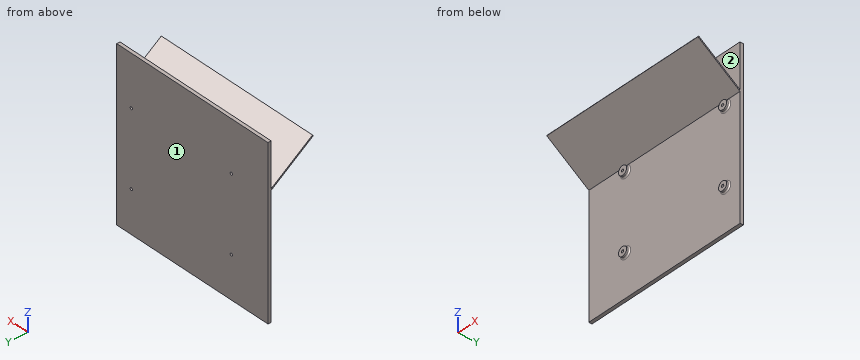
Autodesk Inventor part; units mm, degrees
ref_plane "YZ Plane" through (0, 0, 0) normal (1, 0, 0) x (0, 1, 0)
ref_plane "XZ Plane" through (0, 0, 0) normal (0, 1, 0) x (-1, 0, 0)
ref_plane "XY Plane" through (0, 0, 0) normal (0, 0, 1) x (1, 0, 0)
sketch "Sketch1" plane through (0, 0, 0) normal (0, 1, 0) x (-1, 0, 0)
  line L0 (0, 0) -> (130, 0)
  line L1 (130, 0) -> (130, -130)
  line L2 (130, -130) -> (0, -130)
  line L3 (0, -130) -> (0, 0)
  dimension "d0" = 130
  dimension "d1" = 130
extrude "Extrusion1" add sketch "Sketch1" along normal blind 2.5
sketch "Sketch2" plane through (0, 0, 0) normal (0, -1, 0) x (1, 0, 0)
  line L0 (-2.5, -114.4468) -> (-102.5, -114.4468) construction
  line L1 (-102.5, -114.4468) -> (-102.5, -35.4468) construction
  line L2 (-102.5, -35.4468) -> (-2.5, -35.4468) construction
  line L3 (-2.5, -35.4468) -> (-2.5, -114.4468) construction
  line L4 (-12.5, -97.4468) -> (-98.5, -97.4468) construction
  line L5 (-98.5, -97.4468) -> (-98.5, -39.4468) construction
  line L6 (-98.5, -39.4468) -> (-12.5, -39.4468) construction
  line L7 (-12.5, -39.4468) -> (-12.5, -97.4468) construction
  line L8 (0, 0) -> (-130, 0) construction
  line L9 (-130, -130) -> (0, -130) construction
  line L10 (-130, 0) -> (-130, -130) construction
  circle A0 centre (-12.5, -97.4468) radius 3.5
  circle A1 centre (-98.5, -97.4468) radius 3.5
  circle A2 centre (-12.5, -39.4468) radius 3.5
  circle A3 centre (-98.5, -39.4468) radius 3.5
  line L11 (0, -130) -> (0, 0)
  line L12 (-91.6778, -53.8) -> (-93.3369, -53.8) construction
  line L13 (-93.3369, -53.8) -> (-93.3369, -76.2) construction
  line L14 (-93.3369, -76.2) -> (-91.6778, -76.2) construction
  line L15 (-91.6778, -76.2) -> (-91.6778, -53.8) construction
  dimension "d4" = 86
  dimension "d5" = 58
  dimension "d6" = 100
  dimension "d7" = 79
  dimension "d8" = 4
  dimension "d9" = 4
  dimension "d10" = 130
  dimension "d13" = 7
  dimension "d14" = 7
  dimension "d15" = 7
  dimension "d16" = 7
  dimension "d27" = 2.5
  dimension "d34" = 22.4
  dimension "d35" = 21.2468
  dimension "d36" = 53.8
extrude "Extrusion2" add sketch "Sketch2" along normal blind 2.25
fillet "Fillet1" radius 1 4 edges at (-16, 0, -97.4468) (-16, 0, -39.4468) (-102, 0, -39.4468) (-102, 0, -97.4468)
sketch "Sketch3" plane through (-12.5, -2.25, -97.4468) normal (0, -1, 0) x (1, 0, 0)
  circle A0 centre (0, 0) radius 3.5 construction
  circle A1 centre (-86, 0) radius 3.5 construction
  circle A2 centre (0, 58) radius 3.5 construction
  circle A3 centre (-86, 58) radius 3.5 construction
  circle A4 centre (0, 0) radius 4.5 construction
  circle A5 centre (-86, 58) radius 3.5 construction
  point P0 (12.5, 97.4468)
  point P1 (0, 58)
  point P2 (-86, 58)
  point P3 (-86, 0)
hole "Hole1" at (-12.5, -2.25, -97.4468) at (-12.5, -2.25, -39.4468) at (-98.5, -2.25, -39.4468) at (-98.5, -2.25, -97.4468) direction (0, 1, 0) diameter 2.013 depth 4.75
sketch "Sketch4" plane through (0, 0, 0) normal (1, 0, 0) x (0, 0, -1)
  line L0 (130, 0) -> (0, 0)
  line L1 (35.4468, 0) -> (1.8296, -48.0104) construction
  line L2 (35.4468, 0) -> (12.5038, -32.7661)
  line L3 (12.5038, -32.7661) -> (11.6846, -32.1925)
  line L4 (11.6846, -32.1925) -> (34.2261, 0)
  line L5 (35.4468, 0) -> (34.2261, 0)
  point P0 (35.4468, 0)
  dimension "d28" = 55
  dimension "d29" = 0
  dimension "d30" = 1
  dimension "d31" = 40
extrude "Extrusion3" add sketch "Sketch4" against normal blind 130
sketch "Sketch5" plane through (0, 2.5, 0) normal (1, 0, 0) x (0, 0, -1)
  line L0 (34.2261, -2.5) -> (11.6846, -34.6925)
  point P0 (0, -2.5)
equation "\"d9\" = d8"
equation "\"d14\" = d13"
equation "\"d15\" = d14"
equation "\"d16\" = d15"
equation "\"d36\" = -0.5 * d34 + 0.5 * d10"
properties part number "angle test"
Verification items for the finished model (mm, model axes). Face numbers are marked on the shaded views. A direction names the side the tool comes from. Give positions to 0.01 mm unless a question says otherwise; leave off trailing zeros. Loops run counter-clockwise (first coordinate to the right, second up) from the corner with the lowest first, then second, coordinate; pieces in that order, holes last. Notation, with made-up numbers: (62.25, 81) - (85.25, 81) arc R28 cw to (85.25, 107) - close; hole circle Ø9 at (-23.5, 32.25). An arc over 180 degrees is marked (long way). Write each question's results on one line, items separated by ' | '.
1) Material ranges on L1, parallel to Z at x = -98.5, y = 1.45; L2, parallel to Y at x = -116, z = -95.5; L3, parallel to Y at x = -99, z = -38.5, recorded low to high. Write a range as from..to.
Solution:
L1: -130..-98.45, -96.44..-40.45, -38.44..0 | L2: 0..2.5 | L3: -2.25..2.5
2) Depth check by flat-ended pin: P1, Ø7.5, axis at x = -13, z = -98, coming from the -Y side; P2, Ø1, axis at x = -87.5, y = -9.5, coming from the +Z side; P3, Ø5, axis at x = -63, z = -58, coming from the -Y side; P4, Ø1.2, axis at x = -98.5, z = -39.45, coming from the +Y side. Enter the tip coordinate at first touch or a pass-through.
Solution:
P1: y = -2.25 | P2: z = -27.22 | P3: y = 0 | P4: through
3) Tool access check on the marked faces 1 and 2. Record the directions out of +Z, -Z, +X, -X, +Y, -Y that give a thin tool (end or side, any length) a straight path to the whole face; none if there is none.
Solution:
face 1: +Z, -Z, +X, -X, +Y | face 2: +Z, +X, -X
4) Sectioned sample at B-B on z = -68.5. Record the boundary of the cut face in (x, y).
Solution:
outline: (-130, 0) - (0, 0) - (0, 2.5) - (-130, 2.5) - close
5) Sectioned sample at C-C on y = -12. Record the boundary of the cut face in (x, z).
Solution:
outline: (-130, -27.04) - (0, -27.04) - (0, -25.82) - (-130, -25.82) - close
6) Sectioned sample at A-A on x = -114.5. Record the boundary of the cut face in (y, z).
Solution:
outline: (-32.77, -12.5) - (0, -35.45) - (0, -130) - (2.5, -130) - (2.5, 0) - (0, 0) - (0, -34.23) - (-32.19, -11.68) - close
